Verification items for the finished model (mm, model axes). A direction names the side the tool comes from. Round coordinates to 2 decimals unless told otherwise and drop trailing zeros. Order: outer loops, then holes, each group sorted by start corner. A loop starts at its lowest first (then second) coordinate and runs counter-clockwise, first axis right, second up. Notation, with made-up numbers: (64, 43.25) -> (90, 43.25) arc R9 cw to (90, 53.25) -> close; hole circle Ø6 at (-38, 1). An arc over 180 degrees is marked (long way). Put each result on its own line as item: value.
```python
from build123d import *

# Parameters (mm, degrees)
SKETCH_1_W          = 70
SKETCH_1_H          = 45
EXTRUDE_1_DEPTH     = 3
SKETCH_2_W          = 13
SKETCH_2_H          = 23
CUT_EXTRUDE_1_DEPTH = 10
SKETCH_3_R          = 0.95
CUT_EXTRUDE_2_DEPTH = 10
FILLET_1_R          = 5
FILLET_2_R          = 5
SKETCH_4_R          = 0.95
CUT_EXTRUDE_3_DEPTH = 10
CUT_EXTRUDE_4_DEPTH = 10
SKETCH_9_W          = 65.182596022
SKETCH_9_H          = 39.488918008
EXTRUDE_2_DEPTH     = 40
SKETCH_10_R         = 8
SKETCH_10_W         = 12.58723815
SKETCH_10_H         = 3.324068903
CUT_EXTRUDE_5_DEPTH = 26


with BuildPart() as part:
    # 草图1 → 凸台-拉伸1 (new body)
    with BuildSketch(Plane(origin=(0, 0, 0), x_dir=(1, 0, 0), z_dir=(0, 1, 0))):
        Rectangle(SKETCH_1_W, SKETCH_1_H)
    extrude(amount=EXTRUDE_1_DEPTH)

    # 草图2 → 切除-拉伸1 (cut)
    with BuildSketch(Plane(origin=(0, 3, 0), x_dir=(1, 0, 0), z_dir=(0, 1, 0))):
        with Locations((24, 0)):
            Rectangle(SKETCH_2_W, SKETCH_2_H)
        with Locations((-24, 0)):
            Rectangle(SKETCH_2_W, SKETCH_2_H)
    extrude(amount=-CUT_EXTRUDE_1_DEPTH, mode=Mode.SUBTRACT)

    # 草图3 → 切除-拉伸2 (cut)
    with BuildSketch(Plane(origin=(0, 3, 0), x_dir=(1, 0, 0), z_dir=(0, 1, 0))):
        with Locations((-24, 14)):
            Circle(SKETCH_3_R)
        with Locations((-24, -14)):
            Circle(SKETCH_3_R)
        with Locations((24, 14)):
            Circle(SKETCH_3_R)
        with Locations((24, -14)):
            Circle(SKETCH_3_R)
    extrude(amount=-CUT_EXTRUDE_2_DEPTH, mode=Mode.SUBTRACT)

    # 圆角1
    fillet_1_edges = [part.edges().sort_by_distance(p)[0] for p in [
        (35, 1.5, -22.5),
    ]]
    fillet(fillet_1_edges, radius=FILLET_1_R)

    # 圆角2
    fillet_2_edges = [part.edges().sort_by_distance(p)[0] for p in [
        (35, 1.5, 22.5),
        (-35, 1.5, 22.5),
        (-35, 1.5, -22.5),
    ]]
    fillet(fillet_2_edges, radius=FILLET_2_R)

    # 草图4 → 切除-拉伸3 (cut)
    with BuildSketch(Plane(origin=(0, 3, 0), x_dir=(1, 0, 0), z_dir=(0, 1, 0))):
        with Locations((-30, 17.5)):
            Circle(SKETCH_4_R)
        with Locations((30, 17.5)):
            Circle(SKETCH_4_R)
        with Locations((-30, -17.5)):
            Circle(SKETCH_4_R)
        with Locations((30, -17.5)):
            Circle(SKETCH_4_R)
    extrude(amount=-CUT_EXTRUDE_3_DEPTH, mode=Mode.SUBTRACT)

    # 草图8 → 切除-拉伸4 (cut)
    with BuildSketch(Plane(origin=(0, 3, 0), x_dir=(1, 0, 0), z_dir=(0, 1, 0))):
        with BuildLine():
            Line((-27, 17.5), (27, 17.5))
            ThreePointArc((27, 17.5), (27.878679656, 15.378679656), (30, 14.5))
            Line((30, 14.5), (30, -14.5))
            ThreePointArc((30, -14.5), (27.878679656, -15.378679656), (27, -17.5))
            Line((27, -17.5), (-27, -17.5))
            ThreePointArc((-27, -17.5), (-27.878679656, -15.378679656), (-30, -14.5))
            Line((-30, -14.5), (-30, 14.5))
            ThreePointArc((-30, 14.5), (-27.878679656, 15.378679656), (-27, 17.5))
        make_face()
    extrude(amount=-CUT_EXTRUDE_4_DEPTH, mode=Mode.SUBTRACT)

    # 草图9 → 凸台-拉伸2 (add)
    with BuildSketch(Plane(origin=(0, 3, 0), x_dir=(1, 0, 0), z_dir=(0, 1, 0))):
        with BuildLine():
            Line((-30, -22.5), (30, -22.5))
            ThreePointArc((30, -22.5), (33.535533906, -21.035533906), (35, -17.5))
            Line((35, -17.5), (35, 17.5))
            ThreePointArc((35, 17.5), (33.535533906, 21.035533906), (30, 22.5))
            Line((30, 22.5), (-30, 22.5))
            ThreePointArc((-30, 22.5), (-33.535533906, 21.035533906), (-35, 17.5))
            Line((-35, 17.5), (-35, -17.5))
            ThreePointArc((-35, -17.5), (-33.535533906, -21.035533906), (-30, -22.5))
        make_face()
        Rectangle(SKETCH_9_W, SKETCH_9_H, mode=Mode.SUBTRACT)
    extrude(amount=EXTRUDE_2_DEPTH)

    # 草图10 → 切除-拉伸5 (cut)
    with BuildSketch(Plane.XY.offset(22.5)):
        with Locations((13, 22)):
            Circle(SKETCH_10_R)
        with Locations((-13, 22)):
            Circle(SKETCH_10_R)
        with Locations((0, 7.986881032)):
            Rectangle(SKETCH_10_W, SKETCH_10_H)
    extrude(amount=-CUT_EXTRUDE_5_DEPTH, mode=Mode.SUBTRACT)


solid = part.part
```
Item 1: Tool access check on faces 1 (the face through (6.294, 8, 21)), 2 (the face through (27.86, 1.52, -15.4)), 3 (the face through (35, 21, 0)), 4 (the face through (0, 23, 19.744)). Record the directions out of +Z, -Z, +X, -X, +Y, -Y that give a thin tool (end or side, any length) a straight path to the whole face; none if there is none.
Geometry check:
face 1: +Z
face 2: +Y, -Y
face 3: +Z, -Z, +X, +Y, -Y
face 4: +Y
Item 2: Sectioned sample at D-D, the plane y = 36.5. Record the boundary of the cut face in (x, z), then the cut area to 3 significant figures.
Geometry check:
outline: (-35, -17.5) arc R5 ccw to (-30, -22.5) -> (30, -22.5) arc R5 ccw to (35, -17.5) -> (35, 17.5) arc R5 ccw to (30, 22.5) -> (-30, 22.5) arc R5 ccw to (-35, 17.5) -> close; hole (-32.59, -19.74) -> (32.59, -19.74) -> (32.59, 19.74) -> (-32.59, 19.74) -> close
area: 555 mm2
Item 3: Depth check by flat-ended pin: pin 1 Ø0.8 at (y, z) = (8.5, 20.5) entering from -X; pin 2 Ø8 at (x, z) = (-19.5, -17) entering from -Y; pin 3 Ø2 at (y, z) = (8.5, 21) entering from +X; pin 4 Ø1 at (x, y) = (-19.5, 18.5) entering from +Z. Enter the tip coordinate at first touch or a pass-through.
Geometry check:
pin 1: x = -34.27
pin 2: y = 0
pin 3: x = 34.33
pin 4: z = -19.74
Item 4: Sectioned sample at C-C, the plane x = 13. Record the boundary of the cut face in (y, z).
Geometry check:
outline: (0, -22.5) -> (43, -22.5) -> (43, -19.74) -> (3, -19.74) -> (3, -17.5) -> (0, -17.5) -> close; (0, 17.5) -> (3, 17.5) -> (3, 19.74) -> (14, 19.74) -> (14, 22.5) -> (0, 22.5) -> close; (30, 19.74) -> (43, 19.74) -> (43, 22.5) -> (30, 22.5) -> close
Item 5: Sectioned sample at A-A, the plane x = -1.5. Record the boundary of the cut face in (y, z), then the cut area to 3 significant figures.
Geometry check:
outline: (0, -22.5) -> (43, -22.5) -> (43, -19.74) -> (3, -19.74) -> (3, -17.5) -> (0, -17.5) -> close; (0, 17.5) -> (3, 17.5) -> (3, 19.74) -> (6.32, 19.74) -> (6.32, 22.5) -> (0, 22.5) -> close; (9.65, 19.74) -> (43, 19.74) -> (43, 22.5) -> (9.65, 22.5) -> close
area: 241 mm2
Item 6: Sectioned sample at B-B, the plane y = 22. Record the boundary of the cut face in (x, z).
Geometry check:
outline: (-35, -17.5) arc R5 ccw to (-30, -22.5) -> (30, -22.5) arc R5 ccw to (35, -17.5) -> (35, 17.5) arc R5 ccw to (30, 22.5) -> (21, 22.5) -> (21, 19.74) -> (32.59, 19.74) -> (32.59, -19.74) -> (-32.59, -19.74) -> (-32.59, 19.74) -> (-21, 19.74) -> (-21, 22.5) -> (-30, 22.5) arc R5 ccw to (-35, 17.5) -> close; (-5, 19.74) -> (5, 19.74) -> (5, 22.5) -> (-5, 22.5) -> close
Item 7: Material ranges on line 1 along X through (y, z) = (18.5, -16.5); line 2 along Z through (x, y) = (-4, 39); line 3 along X through (y, z) = (1, 17), recorded low to high.
Geometry check:
line 1: -35 to -32.59, 32.59 to 35
line 2: -22.5 to -19.74, 19.74 to 22.5
line 3: -35 to -30.81, -29.19 to -27.04, 27.04 to 29.19, 30.81 to 35
Item 8: Release check for a two-part mould opening along Z. For faces 5 (the face through (0, 21, -22.5)), 6 (the face through (29.05, 1.52, -17.54)), 7 (the face through (-6.294, 8, 21)) record: pulls with the +Z half, pulls with the -Z half, needs draft (parallel to the pull), parting line crosses it, or undercut.
Geometry check:
face 5: pulls with the -Z half
face 6: undercut
face 7: needs draft
